from build123d import *

# Parameters (mm, degrees)
SKETCH_1_W          = 30
SKETCH_1_H          = 450
EXTRUDE_1_DEPTH     = 30
SKETCH_2_W          = 2
SKETCH_2_H          = 26
CUT_EXTRUDE_1_DEPTH = 452.248268695
SHELL_1_T           = -3
SKETCH_3_R          = 2.55
SKETCH_3_R_2        = 1.6
CUT_EXTRUDE_2_DEPTH = 229.7116088


with BuildPart() as part:
    # 草图1 → 凸台-拉伸1 (new body)
    with BuildSketch(Plane.XY):
        Rectangle(SKETCH_1_W, SKETCH_1_H)
    extrude(amount=EXTRUDE_1_DEPTH)

    # 草图2 → 切除-拉伸1 (cut, through all)
    with BuildSketch(Plane(origin=(0, 225, 0), x_dir=(1, 0, 0), z_dir=(0, 1, 0))):
        with Locations((-14, -15)):
            Rectangle(SKETCH_2_W, SKETCH_2_H)
        with Locations((14, -15)):
            Rectangle(SKETCH_2_W, SKETCH_2_H)
    extrude(amount=-CUT_EXTRUDE_1_DEPTH, mode=Mode.SUBTRACT)

    # 抽壳1
    shell_1_openings = [part.faces().sort_by_distance(p)[0] for p in [
        (0, 225, 15),
        (0, -225, 15),
    ]]
    offset(amount=SHELL_1_T, openings=shell_1_openings)

    # 草图3 → 切除-拉伸2 (cut, through all)
    with BuildSketch(Plane(origin=(13, 0, 0), x_dir=(0, 0, -1), z_dir=(1, 0, 0))):
        with Locations((-15, 188.5)):
            Circle(SKETCH_3_R)
        with Locations((-15, -178.5)):
            Circle(SKETCH_3_R)
        with Locations((-19.5, -220)):
            Circle(SKETCH_3_R_2)
        with Locations((-15, -170.5)):
            Circle(SKETCH_3_R)
        with Locations((-10.5, -220)):
            Circle(SKETCH_3_R_2)
        with BuildLine():
            Line((-20, 205), (-10, 205))
            ThreePointArc((-10, 205), (-15, 210), (-20, 205))
        make_face()
        with BuildLine():
            Line((-20, -195), (-10, -195))
            ThreePointArc((-10, -195), (-15, -200), (-20, -195))
        make_face()
    extrude(amount=-CUT_EXTRUDE_2_DEPTH, mode=Mode.SUBTRACT)


solid = part.part
Can you work these out from the model? Positions are in its coordinate system, mm. A direction names the side the tool comes from. Round coordinates to 2 decimals unless told otherwise and drop trailing zeros. Order: outer loops, then holes, each group sorted by start corner. A loop starts at its lowest first (then second) coordinate and runs counter-clockwise, first axis right, second up. Notation, with made-up numbers: M 33,-7 L 40,-7 A17 ccw 40,15 Z; hole C 50.25,-18.75 d3. An arc over 180 degrees is marked long. Use a Markdown table: item, result.
1) On a 3-axis mill with a long thin cutter (end or side, diameter ignored), from which of +Z, -Z, +X, -X, +Y, -Y can I reach the whole of each face in a straight line? I mean faces 1 (the face through (-11, -225, 14)), 2 (the face through (0, 3, 3)), 3 (the face through (-13, 3, 15)). Say none if no direction works.
Geometry says:
| item | result |
|---|---|
| face 1 | +Z, -Z, +X, -X, -Y |
| face 2 | +Y, -Y |
| face 3 | -X, +Y, -Y |
2) Imagine slicing it at B-B (y = 103). List the corners of the cut face in (x, z) for me, then the cut area to 3 significant figures.
Geometry says:
| item | result |
|---|---|
| outline | M -15,0 L 15,0 L 15,2 L 13,2 L 13,28 L 15,28 L 15,30 L -15,30 L -15,28 L -13,28 L -13,2 L -15,2 Z; hole M -10,3 L 10,3 L 10,27 L -10,27 Z |
| area | 316 mm² |
3) I'm going to push flat-ended pins straight in: P1, Ø2, axis at y = -136, z = 25.5, coming from the +X side; P2, Ø5, axis at y = -220, z = 10.5, coming from the -X side. Where does each tip first touch, or does it pass through?
Geometry says:
| item | result |
|---|---|
| P1 | stops at x = 13 |
| P2 | stops at x = -13 |
4) If we mould it in two halves opening along Z, with no side actions, what happens to faces 4 (the face through (-11, 225, 14)), 5 (the face through (13, 3, 15)), 6 (the face through (0, 3, 0)), 7 (the face through (0, 3, 30))? For each: +Z half, -Z half, draft (parallel to the pull), parting line (faces both ways), or undercut.
Geometry says:
| item | result |
|---|---|
| face 4 | draft |
| face 5 | undercut |
| face 6 | -Z half |
| face 7 | +Z half |
5) Imagine slicing it at A-A (x = 0). List the corners of the cut face in (y, z) for me, then the cut area to 3 significant figures.
Geometry says:
| item | result |
|---|---|
| outline | M -225,0 L 225,0 L 225,3 L -225,3 Z; M -225,27 L 225,27 L 225,30 L -225,30 Z |
| area | 2,700 mm² |
6) If I drill on line 1 along Y through (x, z) = (10.95, 15); line 2 along Z through (x, y) = (12.2, -220); line 3 along Z through (x, y) = (-2.75, -171), over which ranges is the centre line in solid material (lowest first)?
Geometry says:
| item | result |
|---|---|
| line 1 | y = -225 to -200, -195 to -181.05, -175.95 to -173.05, -167.95 to 185.95, 191.05 to 205, 210 to 225 |
| line 2 | z = 0 to 8.9, 12.1 to 17.9, 21.1 to 30 |
| line 3 | z = 0 to 3, 27 to 30 |
